```python
from build123d import *

# Parameters (mm, degrees)
F0_R      = 11
F1_DEPTH  = 14.5
F2_R      = 2.1
F3_DEPTH  = 3.5
F4_R      = 11
F5_DEPTH  = 3.5
F7_DEPTH  = 3.5
F8_R      = 6.5
F9_DEPTH  = 7.34
F10_R     = 0.2032
F11_DEPTH = 25


# Not quite as in the source:
# - a pattern or mirror of a feature is missing from the dataset's text; its kind, count and spacing are read off the source's solid


with BuildPart() as f1:
    # F0 (on Top) → F1 (new body)
    with BuildSketch(Plane.XY):
        Circle(F0_R)
    extrude(amount=F1_DEPTH)

    # F2 (on face) → F3 (join)
    with BuildSketch(Plane(origin=(0, 0, 0), x_dir=(1, 0, 0), z_dir=(0, 0, -1))):
        with BuildLine():
            Line((9.5262794416, 5.5), (3.0310889132, 16.75))
            ThreePointArc((3.0310889132, 16.75), (0, 18.5), (-3.0310889132, 16.75))
            Line((-3.0310889132, 16.75), (-9.5262794416, 5.5))
            ThreePointArc((-9.5262794416, 5.5), (0, 11), (9.5262794416, 5.5))
        make_face()
        with Locations((0, 15)):
            Circle(F2_R, mode=Mode.SUBTRACT)
        with BuildLine():
            ThreePointArc((9.5262794416, -5.5), (0, -11), (-9.5262794416, -5.5))
            Line((-9.5262794416, -5.5), (-3.0310889132, -16.75))
            ThreePointArc((-3.0310889132, -16.75), (0, -18.5), (3.0310889132, -16.75))
            Line((3.0310889132, -16.75), (9.5262794416, -5.5))
        make_face()
        with Locations((0, -15)):
            Circle(F2_R, mode=Mode.SUBTRACT)
    f3 = extrude(amount=-F3_DEPTH)

    # F3_copies: F3 across plane
    add(f3.mirror(Plane(origin=(0, 0, 0), x_dir=(0, 0, -1), z_dir=(-1, 0, 0))))

    # F4 (on face) → F5 (cut)
    with BuildSketch(Plane.XY.offset(3.5)):
        Circle(F4_R)
    extrude(amount=F5_DEPTH, mode=Mode.SUBTRACT)

    # F6 (on face) → F7 (join)
    with BuildSketch(Plane.XY.offset(3.5)):
        Polygon((9.5262794416, 5.5), (0, 11), (-9.5262794416, 5.5), (-9.5262794416, -5.5), (0, -11), (9.5262794416, -5.5), align=None)
    extrude(amount=F7_DEPTH)

    # F8 (on face) → F9 (cut)
    with BuildSketch(Plane(origin=(0, 0, 0), x_dir=(1, 0, 0), z_dir=(0, 0, -1))):
        Circle(F8_R)
    extrude(amount=-F9_DEPTH, mode=Mode.SUBTRACT)

    # F10 (on face) → F11 (join)
    with BuildSketch(Plane.XY.offset(14.5)):
        with Locations((6.7, 0)):
            Circle(F10_R)
        with Locations((6.7, 0.4318)):
            Circle(F10_R)
        with Locations((6.7, -0.4318)):
            Circle(F10_R)
    extrude(amount=F11_DEPTH)


solid = f1.part
```
Input: part model. Units: mm. Frame: model coordinates. A direction names the side the tool comes from. Round coordinates to 2 decimals unless told otherwise and drop trailing zeros. Order: outer loops, then holes, each group sorted by start corner. A loop starts at its lowest first (then second) coordinate and runs counter-clockwise, first axis right, second up. Notation, with made-up numbers: (57.25, 45) - (111.25, 45) arc R31 cw to (111.25, 82) - close; hole circle Ø10 at (65.25, -5). An arc over 180 degrees is marked (long way). Answer in a Markdown table with one row per item.
Item 1: Section query B-B (x = 1). Return the cut outline in (y, z).
Model answer:
| item | result |
|---|---|
| outline | (-18.35, 0) - (-16.85, 0) - (-16.85, 3.5) - (-18.35, 3.5) - close; (-13.15, 0) - (-6.42, 0) - (-6.42, 7.34) - (6.42, 7.34) - (6.42, 0) - (13.15, 0) - (13.15, 3.5) - (10.42, 3.5) - (10.42, 7) - (10.95, 7) - (10.95, 14.5) - (-10.95, 14.5) - (-10.95, 7) - (-10.42, 7) - (-10.42, 3.5) - (-13.15, 3.5) - close; (16.85, 0) - (18.35, 0) - (18.35, 3.5) - (16.85, 3.5) - close |
Item 2: Line query: line 1 (Y direction, x = 0, z = 5.5); line 2 (X direction, y = 0, z = 4); line 3 (X direction, y = -15, z = 0.8). Output: solid intervals per line, ascending.
Model answer:
| item | result |
|---|---|
| line 1 | y = -11 to -6.5, 6.5 to 11 |
| line 2 | x = -9.53 to -6.5, 6.5 to 9.53 |
| line 3 | x = -4.04 to -2.1, 2.1 to 4.04 |
Item 3: Section query D-D (z = 22). Return the cut outline in (x, y).
Model answer:
| item | result |
|---|---|
| outline | circle Ø0.41 at (6.7, -0.43); circle Ø0.41 at (6.7, 0); circle Ø0.41 at (6.7, 0.43) |
Item 4: Section query A-A (y = -15). Return the cut outline in (x, z), then the cut area to 3 significant figures.
Model answer:
| item | result |
|---|---|
| outline | (-4.04, 0) - (-2.1, 0) - (-2.1, 3.5) - (-4.04, 3.5) - close; (2.1, 0) - (4.04, 0) - (4.04, 3.5) - (2.1, 3.5) - close |
| area | 13.6 mm² |
Item 5: Section query C-C (y = 5). Return the cut outline in (x, z), then the cut area to 3 significant figures.
Model answer:
| item | result |
|---|---|
| outline | (-9.8, 0) - (-4.15, 0) - (-4.15, 7.34) - (4.15, 7.34) - (4.15, 0) - (9.8, 0) - (9.8, 3.5) - (9.53, 3.5) - (9.53, 7) - (9.8, 7) - (9.8, 14.5) - (-9.8, 14.5) - (-9.8, 7) - (-9.53, 7) - (-9.53, 3.5) - (-9.8, 3.5) - close |
| area | 221 mm² |
Item 6: Reachability of faces 5 (the flat face through (5, 9, 7)), 6 (the flat face through (0, 12, 3.5)), 7 (the flat face through (0, -12, 3.5)), 8 (the flat face through (-10, 0, 3.5)), 9 (the flat face through (10, 0, 3.5)) from +Z, -Z, +X, -X, +Y, -Y: full face, straight path, thin tool, end or side. Return the list, or none.
Model answer:
| item | result |
|---|---|
| face 5 | +X, +Y |
| face 6 | +Y |
| face 7 | -Y |
| face 8 | -X, +Y, -Y |
| face 9 | +X, +Y, -Y |
Item 7: Pin query (flat end, axial travel): pin 1 (5 mm diameter, centred on y = 10.5, z = 9.5, fed in from +X); pin 2 (3 mm diameter, centred on x = 7, y = -9, fed in from -Z); pin 3 (4 mm diameter, centred on x = -0.5, y = -1, fed in from -Z); pin 4 (8 mm diameter, centred on x = 7, z = 33, fed in from +Y) (3 decimals). Return the tip coordinate at first contact, or that it passes through.
Model answer:
| item | result |
|---|---|
| pin 1 | stops at x = 7.55 |
| pin 2 | stops at z = 0 |
| pin 3 | stops at z = 7.34 |
| pin 4 | stops at y = 0.635 |
Item 8: Mould query, pull axis Y, two halves, no side actions, for faces 1 (the flat face through (0, 0, 7.34)), 2 (the flat face through (9.526, 0, 5)), 3 (the cylindrical face through (-5.158, 3.955, 3.619)), 4 (the flat face through (-6.32, 11.05, 1.73)). Classes: released by +Y, released by -Y, zero draft, split by the parting line, or undercut.
Model answer:
| item | result |
|---|---|
| face 1 | undercut |
| face 2 | zero draft |
| face 3 | undercut |
| face 4 | released by +Y |
